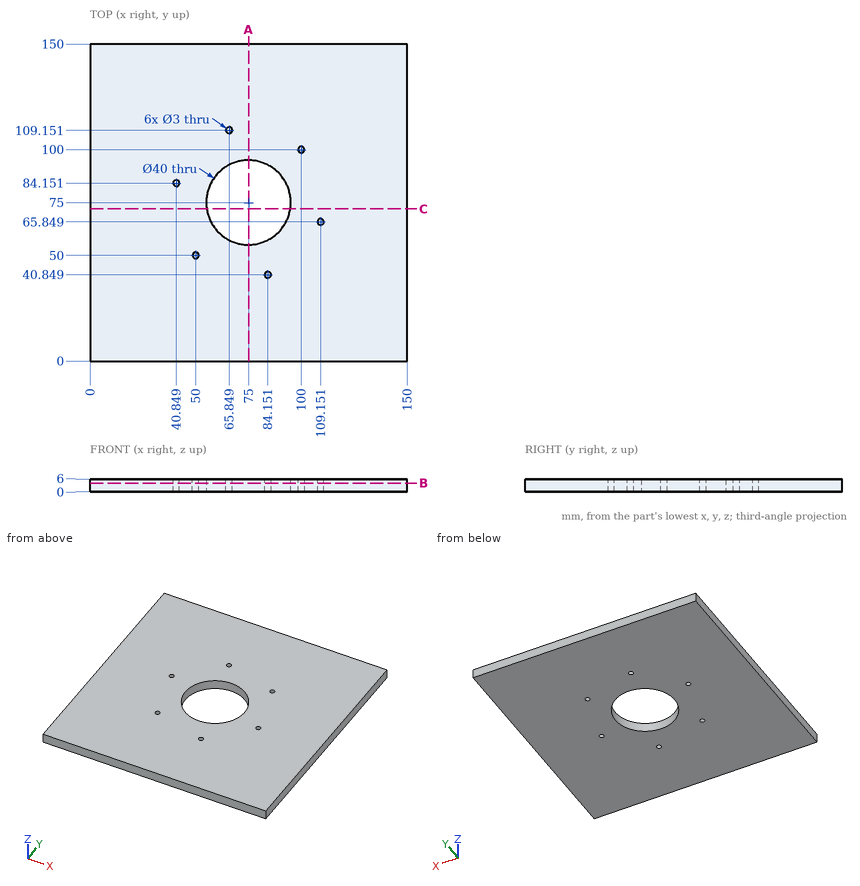
Study the drawing (mm; zero at the part's minimum x, y, z) and answer. Give positions to 0.01 mm unless a question says otherwise; leave off trailing zeros. Write each loop counter-clockwise with the first axis right and the second up, starting at its lowest first coordinate (ties: lowest second). Pieces come first, ordered by that corner, then holes. Notation, with made-up numbers: M 68.5,46 L 81.5,46 A16 ccw 81.5,54 Z; hole C -26,52.5 d6. An arc over 180 degrees is marked long. Put each result on its own line as item: value. Start each with the question number.
1. Consider line 1 along X through (y, z) = (76, 4.25) (1 decimal); line 2 along Y through (x, z) = (100, 4.2). Determine where each line is inside the solid, lowest interval first.
2. The part is cut by section C-C, the plane y = 72. Give the vertices of the cut face in (x, z), and give its area (3 significant figures).
3. The part is cut by section A-A, the plane x = 75. Give the vertices of the cut face in (y, z), and give its area (3 significant figures).
4. The part is cut by section B-B, the plane z = 4.1. Give the vertices of the cut face in (x, y).
Final values:
1. line 1: x = 0 to 55, 95 to 150
1. line 2: y = 0 to 98.5, 101.5 to 150
2. outline: M 0,0 L 55.23,0 L 55.23,6 L 0,6 Z; M 94.77,0 L 150,0 L 150,6 L 94.77,6 Z
2. area: 663 mm²
3. outline: M 0,0 L 55,0 L 55,6 L 0,6 Z; M 95,0 L 150,0 L 150,6 L 95,6 Z
3. area: 660 mm²
4. outline: M 0,0 L 150,0 L 150,150 L 0,150 Z; hole C 40.85,84.15 d3; hole C 50,50 d3; hole C 75,75 d40; hole C 65.85,109.15 d3; hole C 84.15,40.85 d3; hole C 100,100 d3; hole C 109.15,65.85 d3
